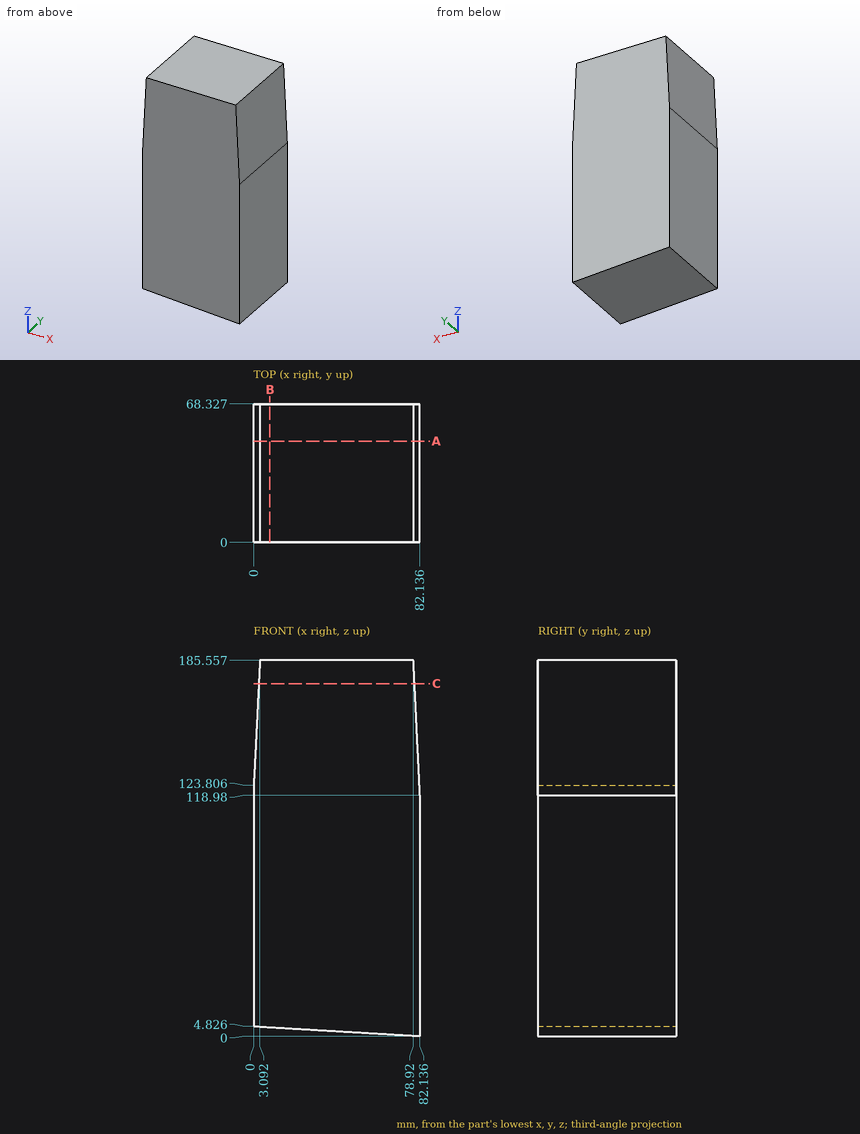
Geometry check sheet. Reference: drawing and pictorial views, mm from the part's lowest x, y, z. Round coordinates to 2 decimals unless told otherwise and drop trailing zeros. Loops run counter-clockwise (first coordinate to the right, second up) from the corner with the lowest first, then second, coordinate; pieces in that order, holes last. Notation, with made-up numbers: (-18, -21.75) -> (37, -21.75) arc R13 cw to (37, -16.75) -> close; hole circle Ø9 at (72.25, 73). An arc over 180 degrees is marked (long way). Answer as a JSON object with one key per item and string values. Group by question number.
Item 1: Cross-section at C-C, the plane z = 174. Record the cut outline in (x, y), plus the area to 3 significant figures.
Item 2: Thickness scan on line 1 along Z through (x, y) = (22, 21); line 2 along Z through (x, y) = (53, 16.5); line 3 along X through (y, z) = (59, 157). Record the ranges inside material, lowest first.
Item 3: Cross-section at A-A, the plane y = 50. Record the cut outline in (x, z), plus the area to 3 significant figures.
Item 4: Cross-section at B-B, the plane x = 8. Record the cut outline in (y, z), plus the area to 3 significant figures.
Item 5: Depth check by flat-ended pin: pin 1 Ø4 at (x, z) = (61.5, 63.5) entering from -Y; pin 2 Ø1.5 at (y, z) = (24, 132) entering from -X; pin 3 Ø1.5 at (x, y) = (10, 38.5) entering from -Z (1 decimal); pin 4 Ø10 at (y, z) = (53.5, 158) entering from -X. Enter the tip coordinate at first touch or a pass-through.
Determined:
{
 "1": {"outline": "(2.51, 0) -> (79.48, 0) -> (79.48, 68.33) -> (2.51, 68.33) -> close", "area": "5,260 mm²"},
 "2": {"line 1": "z = 3.53 to 185.56", "line 2": "z = 1.71 to 185.56", "line 3": "x = 1.66 to 80.3"},
 "3": {"outline": "(0, 4.83) -> (82.14, 0) -> (82.14, 118.98) -> (78.92, 185.56) -> (3.09, 185.56) -> (0, 123.81) -> close", "area": "14,800 mm²"},
 "4": {"outline": "(0, 4.36) -> (68.33, 4.36) -> (68.33, 185.56) -> (0, 185.56) -> close", "area": "12,400 mm²"},
 "5": {"pin 1": "stops at y = 0", "pin 2": "stops at x = 0.37", "pin 3": "stops at z = 4.2", "pin 4": "stops at x = 1.46"}
}
